Can you work these out from the model? Positions are in its coordinate system, mm. A direction names the side the tool comes from. Give positions to 0.01 mm unless a question says otherwise; leave off trailing zeros. Loops run counter-clockwise (first coordinate to the right, second up) from the corner with the lowest first, then second, coordinate; pieces in that order, holes last. Notation, with made-up numbers: (51.5, -8) - (98.5, -8) arc R36 cw to (98.5, 31) - close; hole circle Ø6 at (63, 23). An arc over 180 degrees is marked (long way). Answer as a JSON object with one key per item and string values.
```python
from build123d import *

# Parameters (mm, degrees)
F3_W         = 25
F3_H         = 15
F3_R         = 1.75
F4_DEPTH     = 6
F5_W         = 14
F5_H         = 15
F6_DEPTH     = 6
F7_R         = 5.5
F8_DEPTH     = 1
F9_R         = 1.75
F10_DEPTH    = 2
F11_T1_DEPTH = 15
F11_T3_DEPTH = 45


# Not quite as in the source:
# - a fillet or chamfer that OpenCascade refuses, or shapes differently, is made with other operations: its cross-section is extruded or revolved along the edge and cut away or added


with BuildPart() as f4:
    # F3 (on Front) → F4 (new body)
    with BuildSketch(Plane.XZ):
        with Locations((12.5, 7.5)):
            Rectangle(F3_W, F3_H)
        with Locations((7.5, 7.5)):
            Circle(F3_R, mode=Mode.SUBTRACT)
    extrude(amount=F4_DEPTH)

    # F5 (on face) → F6 (join)
    with BuildSketch(Plane.YZ.offset(25)):
        with Locations((-13, 7.5)):
            Rectangle(F5_W, F5_H)
    extrude(amount=-F6_DEPTH)

    # F7 (on face) → F8 (cut)
    with BuildSketch(Plane.YZ.offset(25)):
        with Locations((-10, 7.5)):
            Circle(F7_R)
    extrude(amount=-F8_DEPTH, mode=Mode.SUBTRACT)

    # F9 (on face) → F10 (cut)
    with BuildSketch(Plane.XZ.offset(6)):
        Polygon((10.9641016151, 7.5), (9.2320508076, 10.5), (5.7679491924, 10.5), (4.0358983849, 7.5), (5.7679491924, 4.5), (9.2320508076, 4.5), align=None)
        with Locations((7.5, 7.5)):
            Circle(F9_R, mode=Mode.SUBTRACT)
    extrude(amount=-F10_DEPTH, mode=Mode.SUBTRACT)

    # F11: fillet of radius 6 on 3 edges, made by hand

    # F11_s2 → F11_t1 (join)
    with BuildSketch(Plane.XY):
        with BuildLine():
            ThreePointArc((13, -6), (17.2426406871, -7.7573593129), (19, -12))
            Line((19, -12), (19, -6))
            Line((19, -6), (13, -6))
        make_face()
    extrude(amount=F11_T1_DEPTH)

    # F11_s4 → F11_t3 (cut)
    with BuildSketch(Plane.XY.offset(-15)):
        with BuildLine():
            ThreePointArc((0, 0), (1.7573593129, -4.2426406871), (6, -6))
            Line((6, -6), (0, -6))
            Line((0, -6), (0, 0))
        make_face()
        with BuildLine():
            ThreePointArc((25, -20), (20.7573593129, -18.2426406871), (19, -14))
            Line((19, -14), (19, -20))
            Line((19, -20), (25, -20))
        make_face()
    extrude(amount=F11_T3_DEPTH, mode=Mode.SUBTRACT)


solid = f4.part
```
1) Imagine slicing it at D-D on z = 4. Write out the boundary of the cut face in (x, y), and give its area (3 significant figures).
Check sheet entries:
{"outline": "(0, 0) arc R6 ccw to (6, -6) - (13, -6) arc R6 cw to (19, -12) - (19, -14) arc R6 ccw to (25, -20) - (25, -14.24) - (24, -14.24) - (24, -5.76) - (25, -5.76) - (25, 0) - close", "area": "218 mm2"}
2) I'm going to push flat-ended pins straight in: P1, Ø3.5, axis at x = 8.5, z = 8, coming from the -Y side; P2, Ø4, axis at y = -12, z = 8.5, coming from the -X side; P3, Ø1, axis at x = 6.5, z = 2, coming from the -Y side. Where does each tip first touch, or does it pass through?
Check sheet entries:
{"P1": "y = -4", "P2": "x = 18.66", "P3": "y = -6"}
3) Which directions (+Z, -Z, +X, -X, +Y, -Y) give clear straight access to the entire face, cutting with the end or side of a thin tool? Please do faces 1 (the cylindrical face through (24.5, -7.5, 2.6)), 2 (the flat face through (10.1, -5, 6)), 3 (the flat face through (19, -13, 8)).
Check sheet entries:
{"face 1": "+X", "face 2": "-Y", "face 3": "+Z, -Z, -X, -Y"}
4) Imagine slicing it at C-C on y = -10. Write out the boundary of the cut face in (x, z), and give its area (3 significant figures).
Check sheet entries:
{"outline": "(18.66, 0) - (25, 0) - (25, 2) - (24, 2) - (24, 13) - (25, 13) - (25, 15) - (18.66, 15) - close", "area": "84.1 mm2"}
5) Imagine slicing it at A-A on x = 7.5. Write out the boundary of the cut face in (y, z), and give its area (3 significant figures).
Check sheet entries:
{"outline": "(-6, 0) - (0, 0) - (0, 5.75) - (-4, 5.75) - (-4, 4.5) - (-6, 4.5) - close; (-6, 10.5) - (-4, 10.5) - (-4, 9.25) - (0, 9.25) - (0, 15) - (-6, 15) - close", "area": "64.0 mm2"}
6) If we mould it in two halves opening along Z, with no side actions, what happens to faces 4 (the flat face through (4.9, -5, 6)), 5 (the cylindrical face through (20.804, -18.289, 7.395)), 6 (the flat face through (15, -5, 15))? For each: released by +Z, released by -Z, zero draft, split by the parting line, or undercut.
Check sheet entries:
{"face 4": "undercut", "face 5": "zero draft", "face 6": "released by +Z"}
7) I need wall thicknesses on L1, parallel to Z at x = 7.5, y = -0.9; L2, parallel to Z at x = 24.5, y = -10; L3, parallel to X at y = -11.75, z = 4.5. Which ranges of each line are inside material? Lowest first, please.
Check sheet entries:
{"L1": "0 to 5.75, 9.25 to 15", "L2": "0 to 2, 13 to 15", "L3": "18.99 to 24"}
8) Imagine slicing it at B-B on z = 6.5. Write out the boundary of the cut face in (x, y).
Check sheet entries:
{"outline": "(0, 0) arc R6 ccw to (4.61, -5.84) - (4.61, -4) - (6.06, -4) - (6.06, 0) - close; (8.94, -4) - (10.39, -4) - (10.39, -6) - (13, -6) arc R6 cw to (19, -12) - (19, -14) arc R6 ccw to (25, -20) - (25, -15.41) - (24, -15.41) - (24, -4.59) - (25, -4.59) - (25, 0) - (8.94, 0) - close"}
